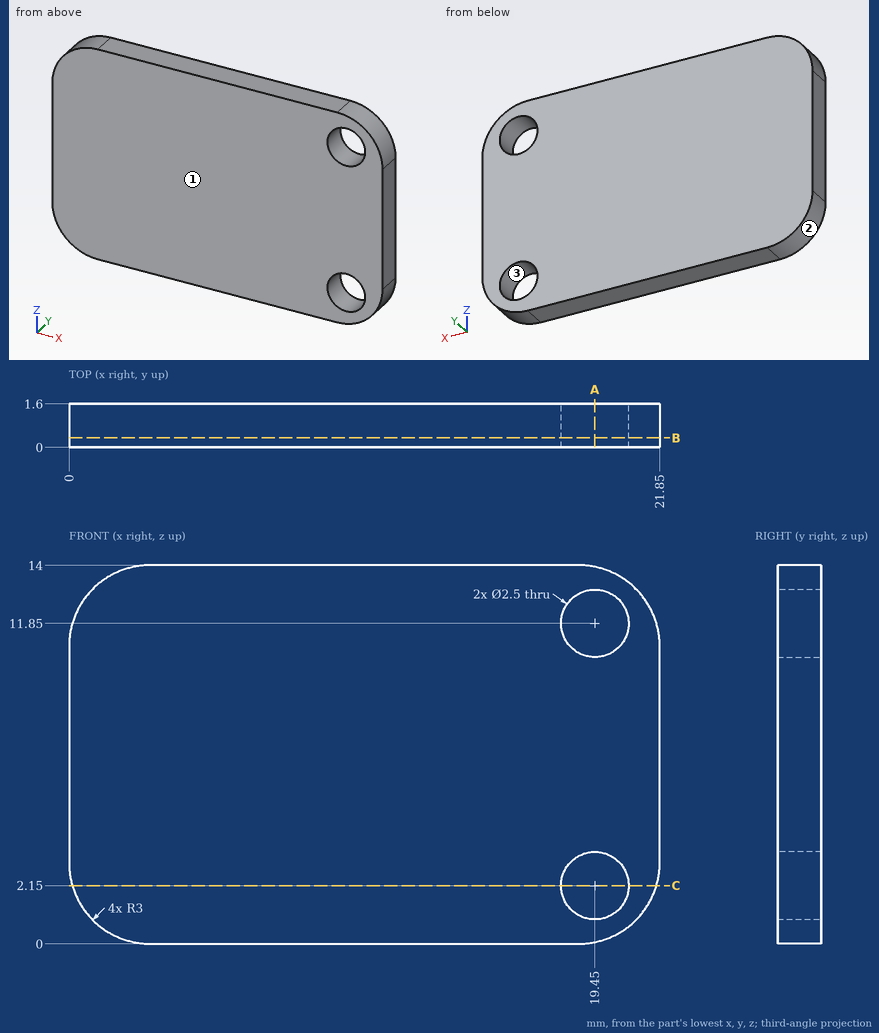
Verification items for this drawing (mm, ordinates from the low corner). Give positions to 0.01 mm unless a question says otherwise; leave off trailing zeros. Loops run counter-clockwise (first coordinate to the right, second up) from the corner with the lowest first, then second, coordinate; pieces in that order, holes last. Notation, with made-up numbers: M 9,11.25 L 32,11.25 A22 ccw 32,41.25 Z; hole C 40.25,-11 d9. An arc over 180 degrees is marked long. Answer as a JSON object with one key per item and string values. Group by question number.
Q1. Material ranges on line 1 along Z through (x, y) = (20, 0.5); line 2 along Z through (x, y) = (19, 0.7); line 3 along X through (y, z) = (0.4, 11.85), recorded low to high. Write a range as [from, to].
Q2. Release check for a two-part mould opening along X. For the marked faces 1, 2 and 3 record: released by +X, released by -X, zero draft, split by the parting line, or undercut.
Q3. Cross-section at C-C on z = 2.15. Record the cut outline in (x, y).
Q4. Cross-section at B-B on y = 0.35. Record the cut outline in (x, z), then the cut area to 3 significant figures.
Q5. Cross-section at A-A on x = 19.45. Record the cut outline in (y, z), then the cut area to 3 significant figures.
Evaluation:
{
 "1": {"line 1": "z = [0.23, 1.03], [3.27, 10.73], [12.97, 13.77]", "line 2": "z = [0, 0.98], [3.32, 10.68], [13.02, 14]", "line 3": "x = [0.12, 18.2], [20.7, 21.73]"},
 "2": {"face 1": "zero draft", "face 2": "released by -X", "face 3": "undercut"},
 "3": {"outline": "M 0.12,0 L 18.2,0 L 18.2,1.6 L 0.12,1.6 Z; M 20.7,0 L 21.73,0 L 21.73,1.6 L 20.7,1.6 Z"},
 "4": {"outline": "M 0,3 A3 ccw 3,0 L 18.85,0 A3 ccw 21.85,3 L 21.85,11 A3 ccw 18.85,14 L 3,14 A3 ccw 0,11 Z; hole C 19.45,2.15 d2.5; hole C 19.45,11.85 d2.5", "area": "288 mm2"},
 "5": {"outline": "M 0,0.06 L 1.6,0.06 L 1.6,0.9 L 0,0.9 Z; M 0,3.4 L 1.6,3.4 L 1.6,10.6 L 0,10.6 Z; M 0,13.1 L 1.6,13.1 L 1.6,13.94 L 0,13.94 Z", "area": "14.2 mm2"}
}
